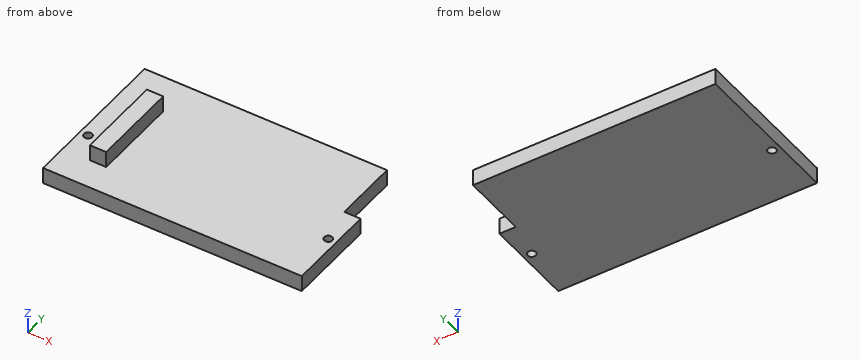
from build123d import *

# Parameters (mm, degrees)
SKETCH1_R           = 1.5
BOSS_EXTRUDE2_DEPTH = 6
SKETCH3_W           = 6
SKETCH3_H           = 32
BOSS_EXTRUDE3_DEPTH = 6


with BuildPart() as part:
    # Sketch1 → Boss-Extrude2 (new body)
    with BuildSketch(Plane.XY):
        Polygon((-47.5, -28.5), (47.5, -28.5), (47.5, 4.5), (41.5, 4.5), (41.5, 28.5), (-47.5, 28.5), align=None)
        with Locations((44.5, -9)):
            Circle(SKETCH1_R, mode=Mode.SUBTRACT)
        with Locations((-44.5, -7.812839041)):
            Circle(SKETCH1_R, mode=Mode.SUBTRACT)
    extrude(amount=BOSS_EXTRUDE2_DEPTH)

    # Sketch3 → Boss-Extrude3 (add)
    with BuildSketch(Plane.XY.offset(6)):
        with Locations((-34.5, -1.5)):
            Rectangle(SKETCH3_W, SKETCH3_H)
    extrude(amount=BOSS_EXTRUDE3_DEPTH)


solid = part.part
Here's how the part is built. I have some questions about the finished solid (model axes, mm). Coordinates: 2 decimals unless noted, no trailing zeros. Order: outer loops, then holes, each group sorted by start corner. A loop starts at its lowest first (then second) coordinate and runs counter-clockwise, first axis right, second up. Notation, with made-up numbers: M 57,49.25 L 72,49.25 A6 cw 72,57.25 Z; hole C 1.25,48.5 d2. An arc over 180 degrees is marked long. Answer as CSV lines item,"result". Start each with the question number.
1. I need wall thicknesses on line 1 (Y direction, x = 44.5, z = 3.5); line 2 (Y direction, x = -44.5, z = 3); line 3 (Z direction, x = -21.5, y = 22). Which ranges of each line are inside material? Lowest first, please. Write a range as [from, to].
2. I want a section at C-C, the plane z = 2.5. Write out the boundary of the cut face in (x, y).
3. I want a section at A-A, the plane x = -44.5. Write out the boundary of the cut face in (y, z), and give its area (3 significant figures).
4. I want a section at B-B, the plane y = 0.5. Write out the boundary of the cut face in (x, z).
5. I want a section at D-D, the plane x = 44.5. Write out the boundary of the cut face in (y, z), and give its area (3 significant figures).
6. For pin 1 (5 mm diameter, centred on y = -5.5, z = 10.5, fed in from -X); pin 2 (1.8 mm diameter, centred on x = -33.5, z = 8, fed in from +Y); pin 3 (3 mm diameter, centred on y = 17.5, z = 2.5, fed in from +X), each with a flat end and sliding along its axis, tell me the tip position at first contact or that it passes through.
Recorded:
1,line 1,"y = [-28.5, -10.5], [-7.5, 4.5]"
1,line 2,"y = [-28.5, -9.31], [-6.31, 28.5]"
1,line 3,"z = [0, 6]"
2,outline,"M -47.5,-28.5 L 47.5,-28.5 L 47.5,4.5 L 41.5,4.5 L 41.5,28.5 L -47.5,28.5 Z; hole C -44.5,-7.81 d3; hole C 44.5,-9 d3"
3,outline,"M -28.5,0 L -9.31,0 L -9.31,6 L -28.5,6 Z; M -6.31,0 L 28.5,0 L 28.5,6 L -6.31,6 Z"
3,area,"324 mm2"
4,outline,"M -47.5,0 L 47.5,0 L 47.5,6 L -31.5,6 L -31.5,12 L -37.5,12 L -37.5,6 L -47.5,6 Z"
5,outline,"M -28.5,0 L -10.5,0 L -10.5,6 L -28.5,6 Z; M -7.5,0 L 4.5,0 L 4.5,6 L -7.5,6 Z"
5,area,"180 mm2"
6,pin 1,"stops at x = -37.5"
6,pin 2,"stops at y = 14.5"
6,pin 3,"stops at x = 41.5"
